Input: part model. Units: mm. Frame: model coordinates. Round coordinates to 2 decimals unless told otherwise and drop trailing zeros. Loops run counter-clockwise (first coordinate to the right, second up) from the corner with the lowest first, then second, coordinate; pieces in that order, holes last.
(1) Cut plane A-A, the plane y = 1.95. Output: boundary loops of the cut face in (x, z).
(2) Line query: line 1 (Z direction, x = -3.25, y = 0.25); line 2 (Z direction, x = 7.75, y = 1.3); line 3 (X direction, y = 0.75, z = -8.25). Output: solid intervals per line, ascending.
(3) Cut plane B-B, the plane y = 2.95. Output: boundary loops of the cut face in (x, z).
(4) First-contact query: pin 1 Ø1 at (x, y) = (1.5, 1.5) entering from +Z. Flat tip, straight axial feed; report the tip coordinate or a pass-through.
Autodesk Inventor part; units mm, degrees
ref_plane "YZ Plane" through (0, 0, 0) normal (1, 0, 0) x (0, 1, 0)
ref_plane "XZ Plane" through (0, 0, 0) normal (0, 1, 0) x (-1, 0, 0)
ref_plane "XY Plane" through (0, 0, 0) normal (0, 0, 1) x (1, 0, 0)
sketch "Sketch1" plane through (0, 0, 0) normal (0, 1, 0) x (-1, 0, 0)
  circle A0 centre (0, 0) radius 10.01
  dimension "d0" = 20.02
extrude "Extrusion1" add sketch "Sketch1" along normal blind 3.5
fillet "Fillet1" radius 1 1 edges at (10.01, 3.5, 0)
fillet "Fillet2" radius 1 1 edges at (10.01, 0, 0)
properties part number "Battery"
Reported:
1. outline: circle Ø20.02 at (0, 0)
2. line 1: z = -9.11 to 9.11
2. line 2: z = -6.34 to 6.34
2. line 3: x = -5.61 to 5.61
3. outline: circle Ø19.81 at (0, 0)
4. pin 1: stops at z = 9.96
